Here's the drawing with two shaded views (mm, measured from the low corner). I have some questions. Round coordinates to 2 decimals unless told otherwise and drop trailing zeros. Loops run counter-clockwise (first coordinate to the right, second up) from the corner with the lowest first, then second, coordinate; pieces in that order, holes last. Notation, with made-up numbers: (18, -16) - (22, -16) arc R31 cw to (22, 23) - close; hole circle Ø6 at (-25.75, 1). An arc over 180 degrees is marked (long way). Use one line per item in the form item = value.
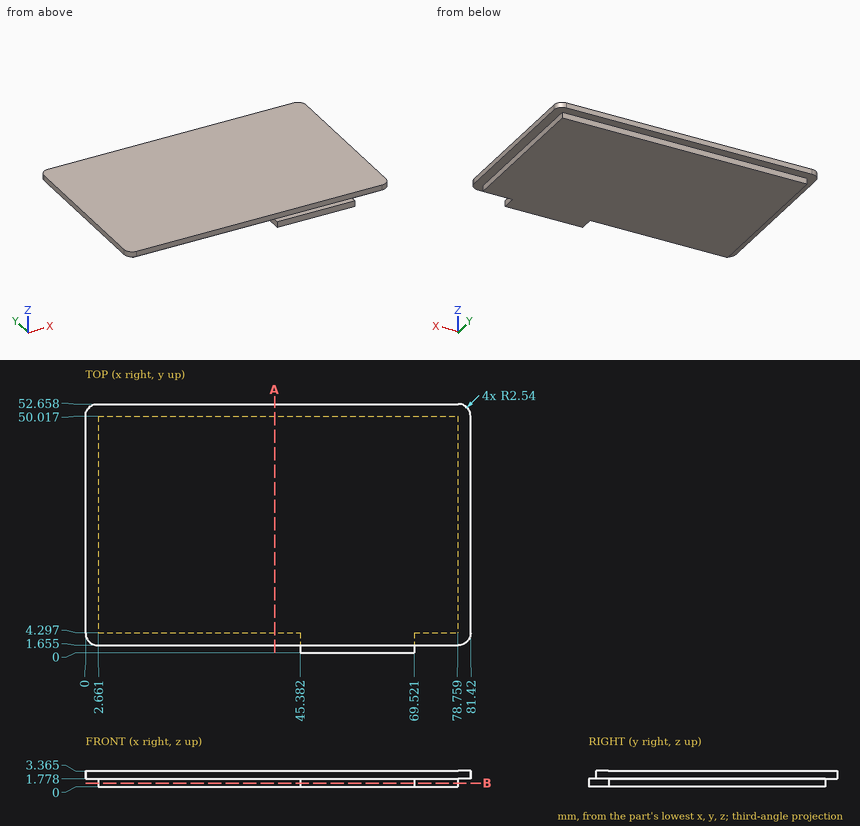
1. Please list where these lines run through material, in increasing order: line 1 along X through (y, z) = (2, 0.45); line 2 along Y through (x, z) = (64, 0.7); line 3 along X through (y, z) = (28.5, 1.7).
Solution:
line_1 = 45.38 to 69.52
line_2 = 0 to 50.02
line_3 = 2.66 to 78.76
2. If we section it at A-A, the plane x = 40: Write out the boundary of the cut face in (y, z) (1 decimal).
Solution:
outline = (1.7, 1.8) - (4.3, 1.8) - (4.3, 0) - (50, 0) - (50, 1.8) - (52.7, 1.8) - (52.7, 3.4) - (1.7, 3.4) - close
3. If we section it at B-B, the plane z = 0.8: Write out the boundary of the cut face in (x, y), plus the area to 3 significant figures.
Solution:
outline = (2.66, 4.3) - (45.38, 4.3) - (45.38, 0) - (69.52, 0) - (69.52, 4.3) - (78.76, 4.3) - (78.76, 50.02) - (2.66, 50.02) - close
area = 3,580 mm^2
4. For P1, Ø0.5, axis at x = 75.5, z = 0.5, coming from the -Y side; P2, Ø1.3, axis at x = 50.5, z = 2.5, coming from the -Y side (1 decimal); P3, Ø0.5, axis at x = 33.5, z = 1, coming from the +Y side; P4, Ø1, axis at x = 72.5, z = 1.5, coming from the +Y side, each with a flat end and sliding along its axis, tell me the tip position at first contact or that it passes through.
Solution:
P1 = 4.3
P2 = 1.7
P3 = 50.02
P4 = 52.66
